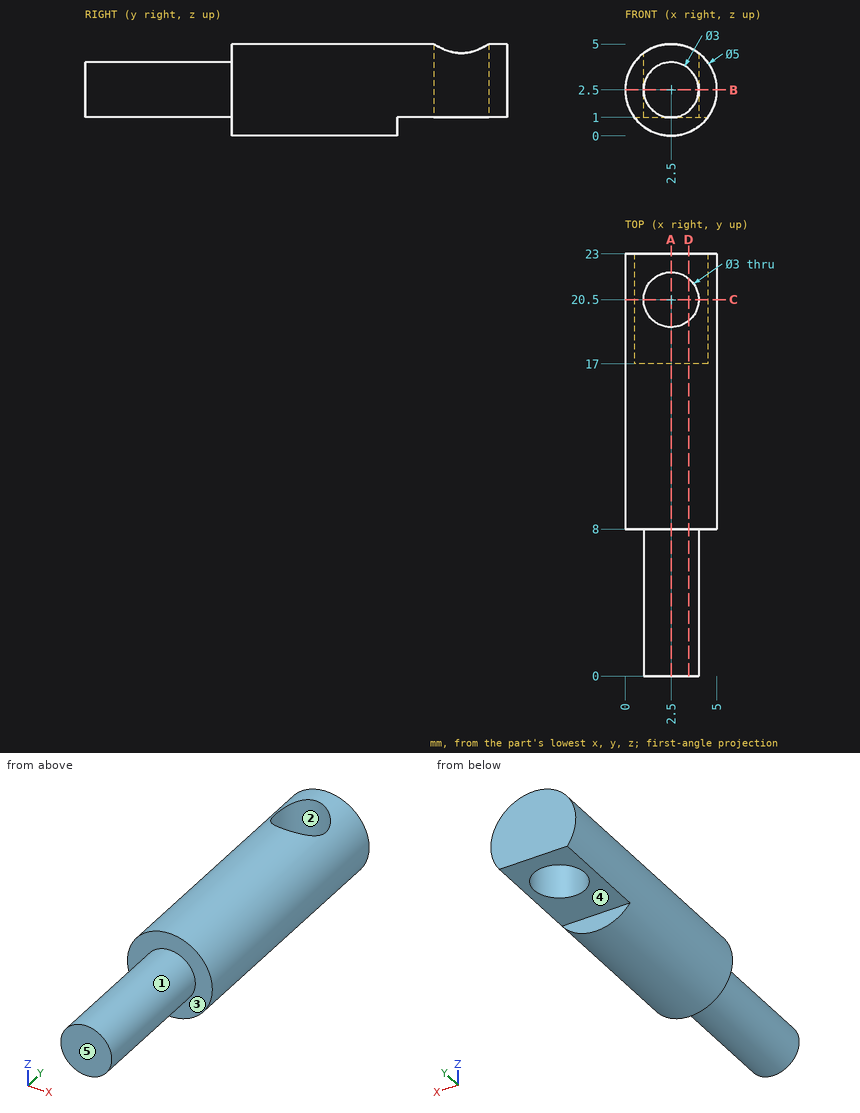
Design review of the part shown in the three views and the two pictorial views. Dimensions are in mm from the part's minimum x, y and z. A direction names the side the tool comes from. Round coordinates to 2 decimals unless told otherwise and drop trailing zeros. Write each loop counter-clockwise with the first axis right and the second up, starting at its lowest first coordinate (ties: lowest second). Pieces come first, ordered by that corner, then holes. Notation, with made-up numbers: M 50.5,69 L 65.5,69 A17 cw 65.5,86 Z; hole C -9,-19 d6. An arc over 180 degrees is marked long. Use a Markdown table: item, result. Add a question column.
Q1. We need section B-B, the plane z = 2.5. State the section outline as (x, y) points.
Q2. We need section A-A, the plane x = 2.5. State the section outline as (y, z) points, plus the area to 3 significant figures.
Q3. The part is to be moulded in two halves that separate along X. For the marked faces 1, 2 and 3, say which applies: pulls with the +X half, pulls with the -X half, needs draft (parallel to the pull), parting line crosses it, or undercut.
Q4. Insertion check: pin 1 (2 mm diameter, centred on x = 1.5, y = 4.5, fed in from -Z); pin 2 (2.5 mm diameter, centred on x = 2.5, y = 20.5, fed in from +Z). Each pin has a flat end and moves straight along its axis. Give the tip position at first contact, or say it passes through.
Q5. To check wall thickness, follow line 1 (Y direction, x = 2.5, z = 3.8); line 2 (Y direction, x = 4.15, z = 0.8); line 3 (X direction, y = 20.5, z = 1.95). State the ranges of each line that lie inside material, in increasing order.
Q6. We need section C-C, the plane y = 20.5. State the section outline as (x, z) points.
Q7. Machinability: for the marked faces 4 and 5, which of the approach directions +Z, -Z, +X, -X, +Y, -Y give a long, thin tool a straight path to every point of the face, cutting with its end or side? Answer none if there is none.
Q8. We need section D-D, the plane x = 3.45. State the section outline as (y, z) points, plus the area to 3 significant figures.
Findings below:
| question | item | result |
|---|---|---|
| 1 | outline | M 0,8 L 1,8 L 1,0 L 4,0 L 4,8 L 5,8 L 5,23 L 0,23 Z; hole C 2.5,20.5 d3 |
| 2 | outline | M 0,1 L 8,1 L 8,0 L 17,0 L 17,1 L 19,1 L 19,5 L 8,5 L 8,4 L 0,4 Z; M 22,1 L 23,1 L 23,5 L 22,5 Z |
| 2 | area | 81.0 mm² |
| 3 | face 1 | parting line crosses it |
| 3 | face 2 | undercut |
| 3 | face 3 | needs draft |
| 4 | pin 1 | stops at z = 1 |
| 4 | pin 2 | passes through |
| 5 | line 1 | y = 0 to 19, 22 to 23 |
| 5 | line 2 | y = 8 to 17 |
| 5 | line 3 | x = 0.06 to 1, 4 to 4.94 |
| 6 | outline | M 0.5,1 L 1,1 L 1,4.5 A2.5 ccw Z; M 4,1 L 4.5,1 A2.5 ccw 4,4.5 Z |
| 7 | face 4 | -Z, +X, -X, +Y |
| 7 | face 5 | +Z, -Z, +X, -X, -Y |
| 8 | outline | M 0,1.34 L 8,1.34 L 8,0.19 L 17,0.19 L 17,1 L 19.34,1 L 19.34,4.81 L 8,4.81 L 8,3.66 L 0,3.66 Z; M 21.66,1 L 23,1 L 23,4.81 L 21.66,4.81 Z |
| 8 | area | 74.2 mm² |
